For this review, take the finished solid that the model builds, in its own axes (mm). Face numbers are marked on the shaded views. Coordinates: 2 decimals unless noted, no trailing zeros. Loops run counter-clockwise (first coordinate to the right, second up) from the corner with the lowest first, then second, coordinate; pieces in that order, holes last. Notation, with made-up numbers: M 31.5,-20 L 62.5,-20 A33 cw 62.5,10 Z; hole C 78.25,-20 d11. An arc over 180 degrees is marked long. Answer as a JSON object with one key per item and string values. Group by question number.
Item 1: Add section B-B (z = 2.35). State the section outline as (x, y) points (3 decimals).
Item 2: Wall thickness on L1, parallel to Y at x = 12.7, z = 1.2 (3 decimals); L2, parallel to X at y = 1.5, z = 1; L3, parallel to Y at x = -1.25, z = 2.8: over which ranges is each line inside the solid? List them lowest first. Write a range as from..to.
Item 3: Insertion check: pin 1 (2 mm diameter, centred on x = 12.7, y = 0, fed in from +Z). The pin has a flat end and moves straight along its axis. Give the tip position at first contact, or say it passes through.
Item 4: Add section A-A (y = 0). State the section outline as (x, z) points (3 decimals).
Item 5: Add section C-C (x = -1.5). State the section outline as (y, z) points, then the cut area to 3 significant figures.
Item 6: Mouldability with a two-part tool opening along X and no side actions: class the marked faces 1, 2, 3 and 4 as +X half, -X half, draft (parallel to the pull), parting line (faces both ways), or undercut.
Item 7: Add section D-D (y = -1.5). State the section outline as (x, z) points, then the cut area to 3 significant figures.
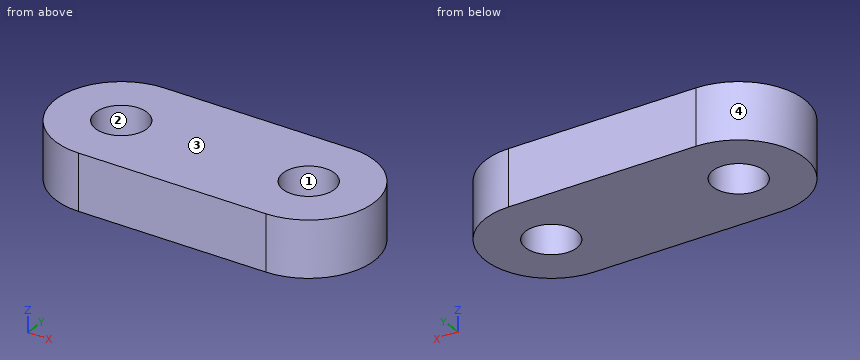
from build123d import *

# Parameters (mm, degrees)
BOSS_EXTRUDE1_DEPTH = 3.81
CUT_EXTRUDE1_START  = -4.81
SKETCH2_R           = 1.7399
CUT_EXTRUDE1_DEPTH  = 5.81


with BuildPart() as part:
    # Sketch1 → Boss-Extrude1 (new body)
    with BuildSketch(Plane.XY):
        with BuildLine():
            Line((0, 4.445), (12.7, 4.445))
            ThreePointArc((12.7, 4.445), (17.145, 0), (12.7, -4.445))
            Line((12.7, -4.445), (0, -4.445))
            ThreePointArc((0, -4.445), (-4.445, 0), (0, 4.445))
        make_face()
    extrude(amount=BOSS_EXTRUDE1_DEPTH)

    # Sketch2 → Cut-Extrude1 (cut)
    with BuildSketch(Plane.XY.offset(3.81).offset(CUT_EXTRUDE1_START)):
        Circle(SKETCH2_R)
    cut_extrude1 = extrude(amount=CUT_EXTRUDE1_DEPTH, mode=Mode.SUBTRACT)

    # Mirror1: Cut-Extrude1 across plane
    add(cut_extrude1.mirror(Plane(origin=(6.35, 0, 0), x_dir=(0, 0, 1), z_dir=(1, 0, 0))), mode=Mode.SUBTRACT)


solid = part.part
From the geometry:
{
 "1": {"outline": "M 0,-4.445 L 12.7,-4.445 A4.445 ccw 12.7,4.445 L 0,4.445 A4.445 ccw Z; hole C 0,0 d3.48; hole C 12.7,0 d3.48"},
 "2": {"L1": "y = -4.445..-1.74, 1.74..4.445", "L2": "x = -4.18..-0.88, 0.88..11.82, 13.58..16.88", "L3": "y = -4.27..-1.21, 1.21..4.27"},
 "3": {"pin 1": "passes through"},
 "4": {"outline": "M -4.445,0 L -1.74,0 L -1.74,3.81 L -4.445,3.81 Z; M 1.74,0 L 10.96,0 L 10.96,3.81 L 1.74,3.81 Z; M 14.44,0 L 17.145,0 L 17.145,3.81 L 14.44,3.81 Z"},
 "5": {"outline": "M -4.18,0 L -0.88,0 L -0.88,3.81 L -4.18,3.81 Z; M 0.88,0 L 4.18,0 L 4.18,3.81 L 0.88,3.81 Z", "area": "25.2 mm²"},
 "6": {"face 1": "undercut", "face 2": "undercut", "face 3": "draft", "face 4": "-X half"},
 "7": {"outline": "M -4.18,0 L -0.88,0 L -0.88,3.81 L -4.18,3.81 Z; M 0.88,0 L 11.82,0 L 11.82,3.81 L 0.88,3.81 Z; M 13.58,0 L 16.88,0 L 16.88,3.81 L 13.58,3.81 Z", "area": "66.8 mm²"}
}
